Part model, mm, in its own coordinate system. A direction names the side the tool comes from. Round coordinates to 2 decimals unless told otherwise and drop trailing zeros. Write each loop counter-clockwise with the first axis right and the second up, starting at its lowest first coordinate (ties: lowest second). Pieces come first, ordered by that corner, then holes. Notation, with made-up numbers: (6, 78) -> (40, 78) arc R16 cw to (40, 109) -> close; hole circle Ø6 at (-34, 31.5). An arc over 180 degrees is marked (long way). Return JSON: item names as keys, results as strings. Group by question number.
(1) Saw through at D-D (z = -9.25). List the corners of the cut face in (x, y).
(2) Tool access for faces 1 (the cylindrical face through (1.88, 1.75, -2.34)), 2 (the cylindrical face through (-2, -1, 0)), 3 (the flat face through (-2, -2, -1)): list every direction of +Z, -Z, +X, -X, +Y, -Y with a clear straight run to the whole face (end or side of a thin tool).
(3) Drill centre lines: L1, parallel to X at y = 0.55, z = 15.25; L2, parallel to Y at x = 1.4, z = -4; L3, parallel to Z at x = 1.55, y = -1.8. Where is each one in solid material? Low to high. Write a range as from..to.
(4) Mould opens along Z. For faces 4 (the flat face through (-2.253, 0.76, 8.299)), 5 (the cylindrical face through (0.02, 0.76, -15.75)), 6 (the flat face through (2.253, 0.76, -8.299)), 7 (the flat face through (1, 0, 1)) say: +Z half, -Z half, draft (parallel to the pull), parting line (faces both ways), or undercut.
(5) Drop flat-ended pins along their axis: pin 1 Ø1.8 at (x, z) = (0, 0) entering from -Y; pin 2 Ø2.5 at (x, z) = (-0.5, -13) entering from +Y; pin 3 Ø1.5 at (x, z) = (-0.5, -6) entering from -Y. Give the stop position or say it passes through.
(6) Saw through at C-C (x = -1.3). List the corners of the cut face in (y, z).
(7) Saw through at A-A (z = 0). List the corners of the cut face in (x, y), plus the area to 3 significant figures.
(8) Saw through at B-B (y = 1.1). State how many separate pieces and enclosed holes the cut face has, plus the area to 3 significant figures.
from build123d import *

# Parameters (mm, degrees)
ESQUISSE1_R                            = 2.9
ESQUISSE1_R_2                          = 2
BOSS_EXTRU_1_DEPTH                     = 2
BOSS_EXTRU_2_START                     = 1.5
ESQUISSE2_R                            = 1
BOSS_EXTRU_2_DEPTH                     = 1.5
ESQUISSE4_R                            = 0.5
ENL_V_MAT_EXTRU_1_DEPTH                = 18.838791999
R_P_TITION_LIN_AIRE1_COUNT             = 4
R_P_TITION_LIN_AIRE1_PITCH             = 2
R_P_TITION_CIRCULAIRE1_COUNT           = 2
R_P_TITION_CIRCULAIRE1_COPY_1_SKETCH_R = 0.5
R_P_TITION_CIRCULAIRE1_COPY_1_DEPTH    = 18.838791999
R_P_TITION_CIRCULAIRE1_COPY_2_SKETCH_R = 0.5
R_P_TITION_CIRCULAIRE1_COPY_2_DEPTH    = 18.838791999
R_P_TITION_CIRCULAIRE1_COPY_3_SKETCH_R = 0.5
R_P_TITION_CIRCULAIRE1_COPY_3_DEPTH    = 18.838791999
BOSS_EXTRU_3_START                     = 0.5
ESQUISSE3_R                            = 3
ESQUISSE3_R_2                          = 2
BOSS_EXTRU_3_DEPTH                     = 0.5


with BuildPart() as part:
    # Esquisse1 → Boss.-Extru.1 (new body)
    with BuildSketch(Plane(origin=(0, 0, 0), x_dir=(1, 0, 0), z_dir=(0, 1, 0))):
        with Locations(Location((0, 0, 0), (0, 0, 270))):
            Circle(ESQUISSE1_R)
        with Locations(Location((0, 0, 0), (0, 0, 270))):
            Circle(ESQUISSE1_R_2, mode=Mode.SUBTRACT)
    extrude(amount=-BOSS_EXTRU_1_DEPTH)

    # Esquisse2 → Boss.-Extru.2 (add)
    with BuildSketch(Plane(origin=(0, 0, 0), x_dir=(1, 0, 0), z_dir=(0, 1, 0)).offset(BOSS_EXTRU_2_START)):
        with BuildLine():
            Line((-1.998691666, 15.322329972), (-2.5, 1.469693846))
            ThreePointArc((-2.5, 1.469693846), (0, -2.9), (2.5, 1.469693846))
            Line((2.5, 1.469693846), (1.998691666, 15.322329972))
            ThreePointArc((1.998691666, 15.322329972), (0, 17.25), (-1.998691666, 15.322329972))
        make_face()
        with Locations(Location((0, 0, 0), (0, 0, 270))):
            Circle(ESQUISSE2_R, mode=Mode.SUBTRACT)
    boss_extru_2 = extrude(amount=-BOSS_EXTRU_2_DEPTH)

    # Esquisse4 → Enlèv. mat.-Extru.1 (cut, through all)
    with BuildSketch(Plane(origin=(0, 1.5, 0), x_dir=(1, 0, 0), z_dir=(0, 1, 0))):
        with Locations(Location((0, 15.25, 0), (0, 0, 270))):
            Circle(ESQUISSE4_R)
    enl_v_mat_extru_1 = extrude(amount=-ENL_V_MAT_EXTRU_1_DEPTH, mode=Mode.SUBTRACT)

    # Répétition linéaire1: Enlèv. mat.-Extru.1 ×4
    with Locations(*[(0, 0, i * R_P_TITION_LIN_AIRE1_PITCH) for i in range(1, R_P_TITION_LIN_AIRE1_COUNT)]):
        add(enl_v_mat_extru_1, mode=Mode.SUBTRACT)

    # Répétition circulaire1: Boss.-Extru.2, Enlèv. mat.-Extru.1 ×2 about axis
    r_p_tition_circulaire1_axis = Axis((0, 0, 0), (0, 1, 0))
    add([boss_extru_2.rotate(r_p_tition_circulaire1_axis, i * 360 / R_P_TITION_CIRCULAIRE1_COUNT) for i in range(1, R_P_TITION_CIRCULAIRE1_COUNT)])
    add([enl_v_mat_extru_1.rotate(r_p_tition_circulaire1_axis, i * 360 / R_P_TITION_CIRCULAIRE1_COUNT) for i in range(1, R_P_TITION_CIRCULAIRE1_COUNT)], mode=Mode.SUBTRACT)

    # Répétition circulaire1 copy 1 sketch → Répétition circulaire1 copy 1 (cut, through all)
    with BuildSketch(Plane(origin=(0, 1.5, -2), x_dir=(-1, 0, 0), z_dir=(0, 1, 0))):
        with Locations(Location((0, 15.25, 0), (0, 0, 270))):
            Circle(R_P_TITION_CIRCULAIRE1_COPY_1_SKETCH_R)
    extrude(amount=-R_P_TITION_CIRCULAIRE1_COPY_1_DEPTH, mode=Mode.SUBTRACT)

    # Répétition circulaire1 copy 2 sketch → Répétition circulaire1 copy 2 (cut, through all)
    with BuildSketch(Plane(origin=(0, 1.5, -4), x_dir=(-1, 0, 0), z_dir=(0, 1, 0))):
        with Locations(Location((0, 15.25, 0), (0, 0, 270))):
            Circle(R_P_TITION_CIRCULAIRE1_COPY_2_SKETCH_R)
    extrude(amount=-R_P_TITION_CIRCULAIRE1_COPY_2_DEPTH, mode=Mode.SUBTRACT)

    # Répétition circulaire1 copy 3 sketch → Répétition circulaire1 copy 3 (cut, through all)
    with BuildSketch(Plane(origin=(0, 1.5, -6), x_dir=(-1, 0, 0), z_dir=(0, 1, 0))):
        with Locations(Location((0, 15.25, 0), (0, 0, 270))):
            Circle(R_P_TITION_CIRCULAIRE1_COPY_3_SKETCH_R)
    extrude(amount=-R_P_TITION_CIRCULAIRE1_COPY_3_DEPTH, mode=Mode.SUBTRACT)

    # Esquisse3 → Boss.-Extru.3 (add)
    with BuildSketch(Plane(origin=(0, 1.5, 0), x_dir=(1, 0, 0), z_dir=(0, 1, 0)).offset(BOSS_EXTRU_3_START)):
        with Locations(Location((0, 0, 0), (0, 0, 33.805876752))):
            Circle(ESQUISSE3_R)
        with Locations(Location((0, 0, 0), (0, 0, 270))):
            Circle(ESQUISSE3_R_2, mode=Mode.SUBTRACT)
    extrude(amount=-BOSS_EXTRU_3_DEPTH)


solid = part.part
Computed values:
{
 "1": {"outline": "(-2.22, 0) -> (-0.5, 0) -> (-0.5, 1.5) -> (-2.22, 1.5) -> close; (0.5, 0) -> (2.22, 0) -> (2.22, 1.5) -> (0.5, 1.5) -> close"},
 "2": {"face 1": "+Y", "face 2": "-Y", "face 3": "+Z, -Z, +X, -X, -Y"},
 "3": {"L1": "-2..-0.5, 0.5..2", "L2": "0..1.5", "L3": "-2.45..-1.26, 1.26..2.45"},
 "4": {"face 4": "+Z half", "face 5": "undercut", "face 6": "-Z half", "face 7": "undercut"},
 "5": {"pin 1": "through", "pin 2": "y = 1.5", "pin 3": "y = 0"},
 "6": {"outline": "(-2, -2.59) -> (0, -2.59) -> (0, -16.77) -> (1.5, -16.77) -> (1.5, -2.7) -> (2, -2.7) -> (2, -1.52) -> (1.5, -1.52) -> (1.5, 1.52) -> (2, 1.52) -> (2, 2.7) -> (1.5, 2.7) -> (1.5, 16.77) -> (0, 16.77) -> (0, 2.59) -> (-2, 2.59) -> (-2, 1.52) -> (0, 1.52) -> (0, -1.52) -> (-2, -1.52) -> close"},
 "7": {"outline": "(-3, 1.5) -> (-2.9, 1.5) -> (-2.9, -2) -> (-2, -2) -> (-2, 0) -> (-1, 0) -> (-1, 1.5) -> (-2, 1.5) -> (-2, 2) -> (-3, 2) -> close; (1, 0) -> (2, 0) -> (2, -2) -> (2.9, -2) -> (2.9, 1.5) -> (3, 1.5) -> (3, 2) -> (2, 2) -> (2, 1.5) -> (1, 1.5) -> close", "area": "10.3 mm2"},
 "8": {"separate pieces": "1", "enclosed holes": "9", "area": "143 mm2"}
}
